```python
from build123d import *

# Parameters (mm, degrees)
F1_DEPTH = 304.8
F2_W     = 12.7
F2_H     = 38.1
F3_DEPTH = 25.4
F4_W     = 12.7
F4_H     = 38.1
F5_DEPTH = 25.4
F6_R     = 4.7625
F7_R     = 2.54
F8_R     = 4.7625


with BuildPart() as f1:
    # F0 (on Right) → F1 (new body)
    with BuildSketch(Plane.YZ):
        Polygon((28.189341, 36.801784), (-22.610659, 36.801784), (-22.610659, 30.451784), (21.839341, 30.451784), (21.839341, -13.998216), (28.189341, -13.998216), align=None)
    extrude(amount=F1_DEPTH)

    # F2 (on face) → F3 (cut)
    with BuildSketch(Plane.XZ.offset(-21.839341)):
        with Locations((6.35, 5.051784)):
            Rectangle(F2_W, F2_H)
    extrude(amount=-F3_DEPTH, mode=Mode.SUBTRACT)

    # F4 (on face) → F5 (cut)
    with BuildSketch(Plane.XZ.offset(-21.839341)):
        with Locations((298.45, 5.051784)):
            Rectangle(F4_W, F4_H)
    extrude(amount=-F5_DEPTH, mode=Mode.SUBTRACT)

    # F6
    f6_edges = [f1.edges().sort_by_distance(p)[0] for p in [
        (152.4, 21.839341, 30.451784),
    ]]
    fillet(f6_edges, radius=F6_R)

    # F7
    f7_edges = [f1.edges().sort_by_distance(p)[0] for p in [
        (152.4, -22.610659, 36.801784),
        (152.4, -22.610659, 30.451784),
        (152.4, 21.839341, -13.998216),
        (152.4, 28.189341, -13.998216),
    ]]
    fillet(f7_edges, radius=F7_R)

    # F8
    f8_edges = [f1.edges().sort_by_distance(p)[0] for p in [
        (292.1, 25.014341, 24.101784),
        (12.7, 25.014341, 24.101784),
    ]]
    fillet(f8_edges, radius=F8_R)


solid = f1.part
```
Read the model definition and answer for the solid it produces. Units are mm, in the model's axes. A direction names the side the tool comes from. Give positions to 0.01 mm unless a question says otherwise; leave off trailing zeros. Write each loop counter-clockwise with the first axis right and the second up, starting at its lowest first coordinate (ties: lowest second). Pieces come first, ordered by that corner, then holes. Notation, with made-up numbers: M -13.5,81 L 39.5,81 A13 ccw 39.5,103 Z; hole C -22,58 d4. An arc over 180 degrees is marked long. Put each result on its own line as item: value. Start each with the question number.
1. The part is cut by section C-C, the plane z = 12.5. Give the vertices of the cut face in (x, y), and give its area (3 significant figures).
2. Which of the six approach directions +Z, -Z, +X, -X, +Y, -Y give full straight-line access (tool end or side, diameter ignored) to faces 1 (the flat face through (304.8, 2, 33)), 2 (the flat face through (301, 25, 24.102)), 3 (the flat face through (150, -2, 30.452)), 4 (the flat face through (12.7, 25, 2))?
3. The part is cut by section B-B, the plane y = -4. Give the vertices of the cut face in (x, z).
4. The part is cut by section A-A, the plane x = 255. Give the vertices of the cut face in (y, z) (1 decimal).
5. Consider line 1 along Y through (x, z) = (117, 12.5); line 2 along Z through (x, y) = (69, 9); line 3 along X through (y, z) = (22.5, 12.5). Determine where each line is inside the solid, lowest interval first.
6. Each of these flat-tipped pins is pushed along its axis until it touches: pin 1 Ø5 at (x, y) = (3, 25.5) entering from -Z; pin 2 Ø4 at (x, z) = (59, 0.5) entering from -Y; pin 3 Ø7 at (y, z) = (26.5, 6.5) entering from +X. Where does it stop, or does it pass through?
Final values:
1. outline: M 12.7,21.84 L 292.1,21.84 L 292.1,28.19 L 12.7,28.19 Z
1. area: 1,770 mm²
2. face 1: +Z, -Z, +X, +Y, -Y
2. face 2: -Z, +X, +Y, -Y
2. face 3: -Z, +X, -X, -Y
2. face 4: -Z, -X, +Y, -Y
3. outline: M 0,30.45 L 304.8,30.45 L 304.8,36.8 L 0,36.8 Z
4. outline: M -22.6,33 A2.5 ccw -20.1,30.5 L 17.1,30.5 A4.8 cw 21.8,25.7 L 21.8,-11.5 A2.5 ccw 24.4,-14 L 25.6,-14 A2.5 ccw 28.2,-11.5 L 28.2,36.8 L -20.1,36.8 A2.5 ccw -22.6,34.3 Z
5. line 1: y = 21.84 to 28.19
5. line 2: z = 30.45 to 36.8
5. line 3: x = 12.7 to 292.1
6. pin 1: stops at z = 24.1
6. pin 2: stops at y = 21.84
6. pin 3: stops at x = 292.1
